Work out the finished part from the listing and answer in its coordinate system (mm). A direction names the side the tool comes from. Coordinates: 2 decimals unless noted, no trailing zeros. Order: outer loops, then holes, each group sorted by start corner. A loop starts at its lowest first (then second) coordinate and runs counter-clockwise, first axis right, second up.
Autodesk Inventor part; units mm, degrees
ref_plane "YZ Plane" through (0, 0, 0) normal (1, 0, 0) x (0, 1, 0)
ref_plane "XZ Plane" through (0, 0, 0) normal (0, 1, 0) x (-1, 0, 0)
ref_plane "XY Plane" through (0, 0, 0) normal (0, 0, 1) x (1, 0, 0)
sketch "Sketch1" plane through (0, 0, 0) normal (1, 0, 0) x (0, 1, 0)
  line L0 (12.7, 0) -> (33.3375, 0)
  line L1 (33.3375, -215.9) -> (12.7, -215.9)
  line L2 (0, -203.2) -> (0, -12.7)
  line L3 (41.275, -14.2875) -> (44.45, -14.2875)
  line L4 (79.375, -49.2125) -> (79.375, -166.6875)
  line L5 (44.45, -201.6125) -> (41.275, -201.6125)
  line L6 (0, -210.6276) -> (0, -5.2724)
  line L7 (33.3375, 0) -> (33.3375, -6.35)
  line L8 (33.3375, -209.55) -> (33.3375, -215.9)
  arc A0 (79.375, -49.2125) -> (44.45, -14.2875) centre (44.45, -49.2125) ccw
  arc A1 (44.45, -201.6125) -> (79.375, -166.6875) centre (44.45, -166.6875) ccw
  arc A2 (33.3375, -6.35) -> (41.275, -14.2875) centre (41.275, -6.35) ccw
  arc A3 (41.275, -201.6125) -> (33.3375, -209.55) centre (41.275, -209.55) ccw
  arc A4 (12.7, 0) -> (0, -12.7) centre (12.7, -12.7) ccw
  arc A5 (0, -203.2) -> (12.7, -215.9) centre (12.7, -203.2) ccw
  point P0 (0, 0)
  point P1 (0, -215.9)
  point P2 (79.375, -201.6125)
  point P3 (79.375, -107.95)
  point P4 (33.3375, -107.95)
  dimension "d0" = 215.9
  dimension "d1" = 79.375
  dimension "d2" = 33.3375
  dimension "d3" = 14.2875
  dimension "d4" = 14.2875
  dimension "d5" = 34.925
  dimension "d6" = 34.925
  dimension "d7" = 7.9375
  dimension "d8" = 12.7
  dimension "d9" = 12.7
extrude "Extrusion1" add sketch "Sketch1" along normal blind 7.9375
sketch "Sketch2" plane through (7.9375, 0, 0) normal (1, 0, 0) x (0, 0, -1)
  line L0 (215.9, 12.7) -> (215.9, 33.3375)
  line L1 (215.9, 33.3375) -> (209.55, 33.3375)
  arc A0 (201.6125, 41.275) -> (209.55, 33.3375) centre (209.55, 41.275) ccw
  line L2 (201.6125, 41.275) -> (201.6125, 44.45)
  arc A1 (201.6125, 44.45) -> (166.6875, 79.375) centre (166.6875, 44.45) ccw
  line L3 (166.6875, 79.375) -> (49.2125, 79.375)
  arc A2 (49.2125, 79.375) -> (14.2875, 44.45) centre (49.2125, 44.45) ccw
  line L4 (14.2875, 44.45) -> (14.2875, 41.275)
  arc A3 (6.35, 33.3375) -> (14.2875, 41.275) centre (6.35, 41.275) ccw
  line L5 (6.35, 33.3375) -> (0, 33.3375)
  line L6 (0, 33.3375) -> (0, 12.7)
  arc A4 (0, 12.7) -> (12.7, 0) centre (12.7, 12.7) ccw
  line L7 (12.7, 0) -> (203.2, 0)
  arc A5 (203.2, 0) -> (215.9, 12.7) centre (203.2, 12.7) ccw
  line L8 (107.95, 79.375) -> (107.95, 0) construction
  point P0 (0, 0)
  point P1 (6.35, 25.4)
  point P2 (52.3875, 39.7002)
  point P3 (107.95, 53.975)
  point P4 (107.95, 39.7002)
  point P5 (209.55, 25.4)
  point P6 (163.5125, 39.7002)
  dimension "d12" = 107.95
  dimension "d13" = 39.7002
  dimension "d15" = 39.7002
  dimension "d16" = 53.975
  dimension "d17" = 52.3875
  dimension "d18" = 6.35
  dimension "d19" = 25.4
sketch "Sketch3" plane through (7.9375, 0, 0) normal (1, 0, 0) x (0, 0, -1)
  line L0 (49.2125, 79.375) -> (166.6875, 79.375) construction
  line L1 (107.95, 79.375) -> (107.95, 0) construction
  point P0 (0, 0)
hole "Hole1" at (7.9375, 39.7002, -107.95) direction (-1, 0, 0) diameter 12.7 depth 25.4 tip angle 118
hole "Hole2" at (7.9375, 53.975, -107.95) direction (-1, 0, 0) diameter 4.9784 depth 25.4 tip angle 118
hole "Hole3" at (7.9375, 25.4, -6.35) at (7.9375, 25.4, -209.55) direction (-1, 0, 0) diameter 4.9784 depth 25.4 tip angle 118
hole "Hole4" at (7.9375, 39.7002, -52.3875) at (7.9375, 39.7002, -163.5125) direction (-1, 0, 0) diameter 6.35 depth 25.4 tip angle 118 countersink diameter 9.525 countersink angle 86
properties part number "Base plate"
1. For faces 4 (the flat face through (4, 33.338, -3)), 5 (the cylindrical face through (3.07, 41.63, -160.99)), determine the directions among +Z, -Z, +X, -X, +Y, -Y from which every point of the face is accessible in a straight line to the end or side of a thin tool.
2. Flat-ended cylindrical pins translate along their axes: pin 1 (1.5 mm diameter, centred on x = 1, y = 64.5, fed in from -Z); pin 2 (4 mm diameter, centred on x = 1, z = -23, fed in from +Y); pin 3 (3 mm diameter, centred on y = 53.975, z = -107.95, fed in from +X); pin 4 (1 mm diameter, centred on x = 5.5, y = 48, fed in from -Z). Find the tip coordinate at first contact, or state that the pin passes through.
3. The part is cut by section B-B (x = 1.5). Count the separate pieces of the cut face and the enclosed holes in it, plus the area to 3 significant figures.
4. The part is cut by section D-D (z = -195.5). Determine the outline of the cut face in (x, y).
5. The part is cut by section A-A (z = -107.95). Determine the outline of the cut face in (x, y) (1 decimal), plus the area to 3 significant figures.
6. Consider probe 1 along Y at (x, z) = (5.25, -107.95) (3 decimals); probe 2 along Y at (x, z) = (6, -209.55); probe 3 along Z at (x, y) = (5.5, 65.5). Determine where each line is inside the solid, lowest interval first.
7. The part is cut by section C-C (y = 5). Determine the outline of the cut face in (x, z), plus the area to 3 significant figures.
8. The mould has two halves that part along Y. Classify faces 1 (the cylindrical face through (3.91, 35.41, -103.27)), 2 (the flat face through (4, 23, -215.9)), 3 (the cylindrical face through (3.913, 68.873, -24.247)): released by +Y, released by -Y, zero draft, split by the parting line, or undercut.
Worked out:
1. face 4: +Z, +X, -X, +Y
1. face 5: +X, -X
2. pin 1: stops at z = -195.8
2. pin 2: stops at y = 69.62
2. pin 3: passes through
2. pin 4: stops at z = -201.48
3. separate pieces: 1
3. enclosed holes: 6
3. area: 15,000 mm2
4. outline: (0, 0) - (7.94, 0) - (7.94, 64.19) - (0, 64.19) - close
5. outline: (0, 0) - (7.9, 0) - (7.9, 33.4) - (0, 33.4) - close; (0, 46.1) - (7.9, 46.1) - (7.9, 51.5) - (0, 51.5) - close; (0, 56.5) - (7.9, 56.5) - (7.9, 79.4) - (0, 79.4) - close
5. area: 490 mm2
6. probe 1: y = 0 to 33.35, 46.05 to 51.486, 56.464 to 79.375
6. probe 2: y = 1.7 to 22.91, 27.89 to 33.34
6. probe 3: z = -194.56 to -21.34
7. outline: (0, -213.3) - (7.94, -213.3) - (7.94, -2.6) - (0, -2.6) - close
7. area: 1,670 mm2
8. face 1: undercut
8. face 2: zero draft
8. face 3: released by +Y
